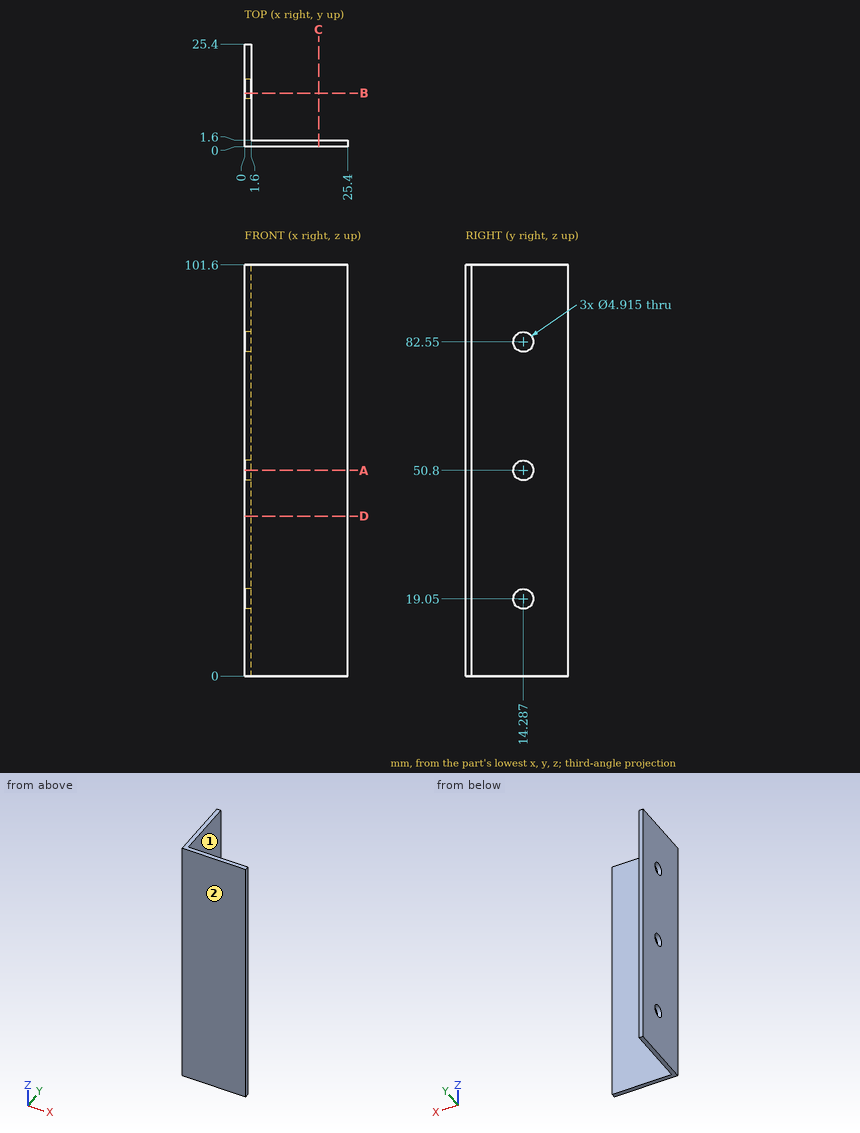
Geometry check sheet. Reference: drawing and pictorial views, mm from the part's lowest x, y, z. A direction names the side the tool comes from. Round coordinates to 2 decimals unless told otherwise and drop trailing zeros. Write each loop counter-clockwise with the first axis right and the second up, starting at its lowest first coordinate (ties: lowest second). Pieces come first, ordered by that corner, then holes.
(1) Material ranges on line 1 (Y direction, x = 1.05, z = 19.05) (1 decimal); line 2 (Y direction, x = 10.25, z = 79), recorded low to high.
Returned:
line 1: y = 0 to 11.8, 16.7 to 25.4
line 2: y = 0 to 1.6
(2) Section check A-A (z = 50.8). Enter the section's corners in (x, y) (1 decimal).
Returned:
outline: (0, 0) - (25.4, 0) - (25.4, 1.6) - (1.6, 1.6) - (1.6, 11.8) - (0, 11.8) - close; (0, 16.7) - (1.6, 16.7) - (1.6, 25.4) - (0, 25.4) - close
(3) Section check C-C (x = 18.25). Enter the section's corners in (y, z).
Returned:
outline: (0, 0) - (1.6, 0) - (1.6, 101.6) - (0, 101.6) - close
(4) Access from +Z, -Z, +X, -X, +Y, -Y to the whole of each face (thin tool, end or side, straight path). Record for the marked faces 1 and 2.
Returned:
face 1: +Z, -Z, +X, +Y
face 2: +Z, -Z, +X, -X, -Y
(5) Depth check by flat-ended pin: pin 1 Ø4 at (y, z) = (14.29, 82.55) entering from -X; pin 2 Ø12 at (x, z) = (17, 13.5) entering from +Y; pin 3 Ø6.5 at (y, z) = (14.29, 50.8) entering from +X. Enter the tip coordinate at first touch or a pass-through.
Returned:
pin 1: passes through
pin 2: stops at y = 1.6
pin 3: stops at x = 1.6
(6) Section check D-D (z = 39.5). Enter the section's corners in (x, y).
Returned:
outline: (0, 0) - (25.4, 0) - (25.4, 1.6) - (1.6, 1.6) - (1.6, 25.4) - (0, 25.4) - close
(7) Section check B-B (y = 13.25). Enter the section's corners in (x, z).
Returned:
outline: (0, 0) - (1.6, 0) - (1.6, 16.82) - (0, 16.82) - close; (0, 21.28) - (1.6, 21.28) - (1.6, 48.57) - (0, 48.57) - close; (0, 53.03) - (1.6, 53.03) - (1.6, 80.32) - (0, 80.32) - close; (0, 84.78) - (1.6, 84.78) - (1.6, 101.6) - (0, 101.6) - close
